Autodesk Inventor part; units mm, degrees
ref_plane "YZ Plane" through (0, 0, 0) normal (1, 0, 0) x (0, 1, 0)
ref_plane "XZ Plane" through (0, 0, 0) normal (0, 1, 0) x (-1, 0, 0)
ref_plane "XY Plane" through (0, 0, 0) normal (0, 0, 1) x (1, 0, 0)
sketch "Sketch1" plane through (0, 0, 0) normal (0, 0, 1) x (1, 0, 0)
  line L0 (0, 0) -> (-210, 0)
  line L1 (-210, 0) -> (-210, 200)
  line L2 (-210, 200) -> (0, 200)
  line L3 (0, 200) -> (0, 0)
  line L4 (-65.5, 79) -> (-65.5, 170)
  line L5 (-65.5, 170) -> (0, 170)
  line L6 (-65.5, 79) -> (-20, 79)
  line L7 (-20, 79) -> (-20, 129)
  line L8 (-20, 129) -> (0, 129)
  line L9 (0, 129) -> (0, 170)
  point P0 (0, 149.5)
  point P1 (0, 129)
  dimension "d0" = 210
  dimension "d1" = 200
  dimension "d2" = 91
  dimension "d3" = 45.5
  dimension "d4" = 50
  dimension "d5" = 20
  dimension "d6" = 30
extrude "Extrusion1" add sketch "Sketch1" along normal blind 9.653 contours L0 L1 L2 L3 L5 L4 L6 L7 L8
sketch "Sketch2" plane through (0, 0, 9.653) normal (0, 0, 1) x (1, 0, 0)
  point P0 (0, 0)
properties part number "base1ek"
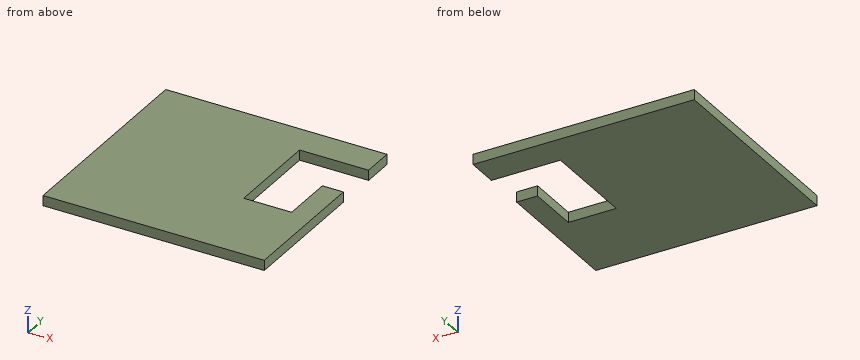
Design review of the part built by this model. Coordinates are the model's own, in mm. Give positions to 0.01 mm unless a question says otherwise; leave off trailing zeros. Loops run counter-clockwise (first coordinate to the right, second up) from the corner with the lowest first, then second, coordinate; pieces in that order, holes last. Notation, with made-up numbers: M -0.5,57 L 37.5,57 A29 cw 37.5,77 Z; hole C 86.25,79.5 d10. An arc over 180 degrees is marked long. Return JSON: item names as keys, results as strings. Group by question number.
Item 1: We need section C-C (z = 5). Give the boundary of the cut face in (x, y).
Item 2: We need section A-A (y = 96). Give the boundary of the cut face in (x, z).
Item 3: We need section B-B (x = -14). Give the boundary of the cut face in (y, z), and give its area (3 significant figures).
Item 4: We need section D-D (y = 167). Give the boundary of the cut face in (x, z), and give its area (3 significant figures).
Item 5: For probe 1 along Y at (x, z) = (-26.5, 8.5); probe 2 along X at (y, z) = (104, 2.75); probe 3 along X at (y, z) = (139, 9), list the stretches that pass through material, from the lowest coordinate up.
Output:
{
 "1": {"outline": "M -210,0 L 0,0 L 0,129 L -20,129 L -20,79 L -65.5,79 L -65.5,170 L 0,170 L 0,200 L -210,200 Z"},
 "2": {"outline": "M -210,0 L -65.5,0 L -65.5,9.65 L -210,9.65 Z; M -20,0 L 0,0 L 0,9.65 L -20,9.65 Z"},
 "3": {"outline": "M 0,0 L 129,0 L 129,9.65 L 0,9.65 Z; M 170,0 L 200,0 L 200,9.65 L 170,9.65 Z", "area": "1,530 mm^2"},
 "4": {"outline": "M -210,0 L -65.5,0 L -65.5,9.65 L -210,9.65 Z", "area": "1,390 mm^2"},
 "5": {"probe 1": "y = 0 to 79, 170 to 200", "probe 2": "x = -210 to -65.5, -20 to 0", "probe 3": "x = -210 to -65.5"}
}
